Can you work these out from the model? Positions are in its coordinate system, mm. A direction names the side the tool comes from. Coordinates: 2 decimals unless noted, no trailing zeros. Loops run counter-clockwise (first coordinate to the right, second up) from the corner with the lowest first, then second, coordinate; pieces in that order, holes last.
```python
from build123d import *

# Parameters (mm, degrees)
SKETCH1_W           = 34
SKETCH1_H           = 27.5
SKETCH1_R           = 1.75
BOSS_EXTRUDE1_DEPTH = 5
FILLET1_R           = 2
SKETCH2_R           = 5.25
CUT_EXTRUDE1_DEPTH  = 0.4


with BuildPart() as part:
    # Sketch1 → Boss-Extrude1 (new body)
    with BuildSketch(Plane(origin=(0, 0, 0), x_dir=(1, 0, 0), z_dir=(0, 1, 0))):
        Rectangle(SKETCH1_W, SKETCH1_H)
        with Locations(Location((0, 8.75, 0), (0, 0, 270))):
            Circle(SKETCH1_R, mode=Mode.SUBTRACT)
        with Locations(Location((-11, -2.75, 0), (0, 0, 270))):
            Circle(SKETCH1_R, mode=Mode.SUBTRACT)
        with Locations(Location((11, -2.75, 0), (0, 0, 270))):
            Circle(SKETCH1_R, mode=Mode.SUBTRACT)
    extrude(amount=BOSS_EXTRUDE1_DEPTH)

    # Fillet1
    fillet1_edges = [part.edges().sort_by_distance(p)[0] for p in [
        (-17, 5, 0),
        (17, 5, 0),
    ]]
    fillet(fillet1_edges, radius=FILLET1_R)

    # Sketch2 → Cut-Extrude1 (cut)
    with BuildSketch(Plane.XZ):
        with Locations(Location((-5.3, 7.5, 0), (0, 0, 270))):
            Circle(SKETCH2_R)
        with Locations(Location((5.3, 7.5, 0), (0, 0, 270))):
            Circle(SKETCH2_R)
        with Locations(Location((0, -1.7, 0), (0, 0, 270))):
            Circle(SKETCH2_R)
    extrude(amount=-CUT_EXTRUDE1_DEPTH, mode=Mode.SUBTRACT)


solid = part.part
```
(1) If I drill on probe 1 along X at (y, z) = (2.3, 2.75); probe 2 along Y at (x, z) = (3, 8.5); probe 3 along X at (y, z) = (3.8, -9.5), over which ranges is the centre line in solid material (lowest first)?
Check values:
probe 1: x = -17 to -12.75, -9.25 to 9.25, 12.75 to 17
probe 2: y = 0.4 to 5
probe 3: x = -16.83 to -1.58, 1.58 to 16.83
(2) I want a section at C-C on z = 1.75. Write out the boundary of the cut face in (x, y).
Check values:
outline: (-17, 0) - (-12.44, 0) - (-12.44, 5) - (-15, 5) arc R2 ccw to (-17, 3) - close; (-9.56, 0) - (-3.96, 0) - (-3.96, 0.4) - (3.96, 0.4) - (3.96, 0) - (9.56, 0) - (9.56, 5) - (-9.56, 5) - close; (12.44, 0) - (17, 0) - (17, 3) arc R2 ccw to (15, 5) - (12.44, 5) - close
(3) I want a section at B-B on y = 2.55. Write out the boundary of the cut face in (x, z).
Check values:
outline: (-17, -13.75) - (17, -13.75) - (17, 13.75) - (-17, 13.75) - close; hole circle Ø3.5 at (-11, 2.75); hole circle Ø3.5 at (0, -8.75); hole circle Ø3.5 at (11, 2.75)
(4) I want a section at A-A on x = -11. Write out the boundary of the cut face in (y, z), then the cut area to 3 significant figures.
Check values:
outline: (0, -13.75) - (5, -13.75) - (5, 1) - (0, 1) - close; (0, 4.5) - (5, 4.5) - (5, 13.75) - (0, 13.75) - close
area: 120 mm2
(5) I'm going to push flat-ended pins straight in: pin 1 (1.5 mm diameter, centred on y = 4.5, z = -6.5, fed in from -X); pin 2 (2 mm diameter, centred on x = 11, z = 2.75, fed in from -Y). Where does each tip first touch, or does it pass through?
Check values:
pin 1: stops at x = -16.85
pin 2: passes through
(6) Which directions (+Z, -Z, +X, -X, +Y, -Y) give clear straight access to the entire face, cutting with the end or side of a thin tool? Please do faces 1 (the cylindrical face through (-7.31, 0.2, 2.65)), 2 (the flat face through (-4, 0, -6)).
Check values:
face 1: -Y
face 2: +Z, -Z, +X, -X, -Y
(7) If we mould it in two halves opening along X, with no side actions, what happens to faces 3 (the cylindrical face through (-0.67, 2.465, -7.133)), 4 (the cylindrical face through (16.43, 4.4, -0.19)), 5 (the flat face through (0, 2, -13.75))? For each: released by +X, released by -X, zero draft, split by the parting line, or undercut.
Check values:
face 3: undercut
face 4: released by +X
face 5: zero draft
(8) I want a section at D-D on z = -9. Write out the boundary of the cut face in (x, y), then the cut area to 3 significant figures.
Check values:
outline: (-17, 0) - (-1.73, 0) - (-1.73, 5) - (-15, 5) arc R2 ccw to (-17, 3) - close; (1.73, 0) - (17, 0) - (17, 3) arc R2 ccw to (15, 5) - (1.73, 5) - close
area: 151 mm2
